Source: three-view drawing plus pictorial views. Frame: mm from the lowest corner of the part. A direction names the side the tool comes from. Give positions to 0.01 mm unless a question says otherwise; leave off trailing zeros. Order: outer loops, then holes, each group sorted by start corner. A loop starts at its lowest first (then second) coordinate and runs counter-clockwise, first axis right, second up. Notation, with made-up numbers: (67, 61) -> (73, 61) arc R20 ccw to (73, 91) -> close; hole circle Ø1 at (47.5, 4.25). An arc over 180 degrees is marked (long way). Answer in a Markdown table with one row per item. Add a question column.
Q1. Cut plane B-B on y = 63.5. Return the cut outline in (x, z) (3 decimals), and give its area (3 significant figures).
Q2. Cut plane C-C on z = 263.5. Return the cut outline in (x, y), and give its area (3 significant figures).
Q3. Pull-direction query (Z, two-part tool) for the marked faces 1, 2 and 3; classes: +Z half, -Z half, draft (parallel to the pull), parting line (faces both ways), or undercut.
Q4. Set-up query: the marked faces 4 and 5. Return all of +Z, -Z, +X, -X, +Y, -Y with unobstructed straight access to the full face (end or side cutting, diameter ignored); none if empty.
Q5. Line query: line 1 along Z through (x, y) = (40.5, 83); line 2 along Y through (x, z) = (64, 310.5); line 3 along Z through (x, y) = (56.5, 113). Output: solid intervals per line, ascending. Write a range as from..to.
Q6. Cut plane A-A on x = 33. Return the cut outline in (y, z), and give its area (3 significant figures).
Q7. Contact query for flat-ended pins moving along their axis: P1, Ø10, axis at x = 47, y = 29.5, coming from the +Z side; P2, Ø10, axis at x = 68, z = 322, coming from the +Y side; P3, Ø3, axis at x = 65.5, z = 304, coming from the -Y side. Output: stop coordinate, or through.
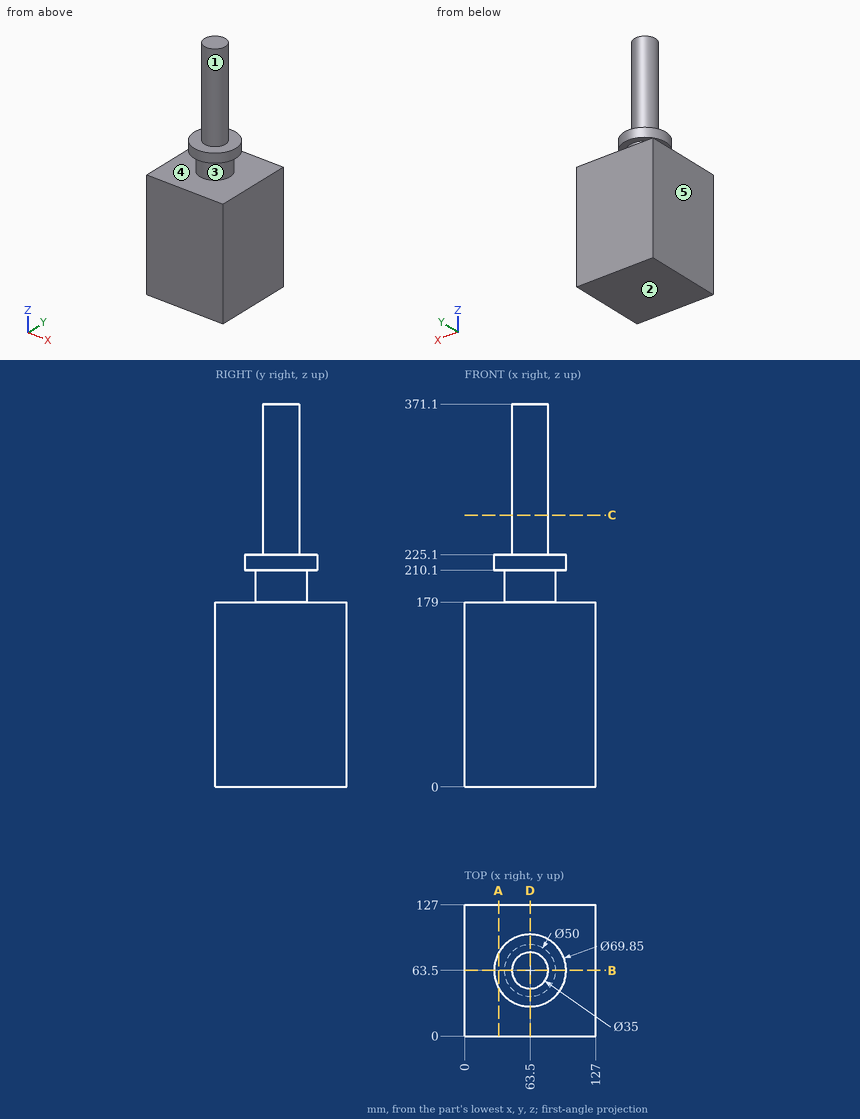
Completed:
| question | item | result |
|---|---|---|
| 1 | outline | (0, 0) -> (127, 0) -> (127, 179) -> (88.5, 179) -> (88.5, 210.1) -> (98.425, 210.1) -> (98.425, 225.1) -> (81, 225.1) -> (81, 371.1) -> (46, 371.1) -> (46, 225.1) -> (28.575, 225.1) -> (28.575, 210.1) -> (38.5, 210.1) -> (38.5, 179) -> (0, 179) -> close |
| 1 | area | 30,400 mm² |
| 2 | outline | circle Ø35 at (63.5, 63.5) |
| 2 | area | 962 mm² |
| 3 | face 1 | draft |
| 3 | face 2 | -Z half |
| 3 | face 3 | undercut |
| 4 | face 4 | none |
| 4 | face 5 | +Z, -Z, -X, +Y, -Y |
| 5 | line 1 | z = 0..179, 210.1..225.1 |
| 5 | line 2 | y = 46.01..80.99 |
| 5 | line 3 | z = 0..179 |
| 6 | outline | (0, 0) -> (127, 0) -> (127, 179) -> (0, 179) -> close; (46.49, 210.1) -> (80.51, 210.1) -> (80.51, 225.1) -> (46.49, 225.1) -> close |
| 6 | area | 23,200 mm² |
| 7 | P1 | stops at z = 225.1 |
| 7 | P2 | stops at y = 81 |
| 7 | P3 | stops at y = 46.01 |
